```python
from build123d import *

# Parameters (mm, degrees)
BOSS_EXTRUDE1_DEPTH = 40
SKETCH3_R           = 1.5
CUT_EXTRUDE2_DEPTH  = 1
SKETCH4_R           = 1.5
SKETCH4_R_2         = 6
CUT_EXTRUDE3_DEPTH  = 10


with BuildPart() as part:
    # Sketch1 → Boss-Extrude1 (new body)
    with BuildSketch(Plane.XY):
        Polygon((0, 13), (0, 14), (7, 14), (11, 7.07179677), (10.133974596, 6.57179677), (6.422649731, 13), (1, 13), align=None)
    extrude(amount=BOSS_EXTRUDE1_DEPTH)

    # Sketch3 → Cut-Extrude2 (cut)
    with BuildSketch(Plane(origin=(11.312177826, 6.531088913, 0), x_dir=(0, 0, -1), z_dir=(0.8660254037844402, 0.4999999999999976, 0))):
        with Locations(Location((-36, 4.624355653, 0), (0, 0, 90))):
            Circle(SKETCH3_R)
        with Locations(Location((-4, 4.624355653, 0), (0, 0, 90))):
            Circle(SKETCH3_R)
        Polygon((-33.701530723, 0.624355653), (-27.721710311, 7.927360795), (-12.278289689, 7.927360795), (-6.298469277, 0.624355653), align=None)
    extrude(amount=-CUT_EXTRUDE2_DEPTH, mode=Mode.SUBTRACT)

    # Sketch4 → Cut-Extrude3 (cut)
    with BuildSketch(Plane(origin=(0, 14, 0), x_dir=(-1, 0, 0), z_dir=(0, 1, 0))):
        with Locations(Location((-3, 24.5, 0), (0, 0, 90))):
            Circle(SKETCH4_R)
        with Locations((4.185654705, 10)):
            Circle(SKETCH4_R_2)
        with Locations((4.185654705, 39)):
            Circle(SKETCH4_R_2)
    extrude(amount=-CUT_EXTRUDE3_DEPTH, mode=Mode.SUBTRACT)


solid = part.part
```
Source: CAD feature listing. Evaluate the final solid. Frame: model axes, mm. A direction names the side the tool comes from. Give positions to 0.01 mm unless a question says otherwise; leave off trailing zeros. Order: outer loops, then holes, each group sorted by start corner. A loop starts at its lowest first (then second) coordinate and runs counter-clockwise, first axis right, second up. Notation, with made-up numbers: (12, 10.5) -> (61, 10.5) arc R30 ccw to (61, 45.5) -> close; hole circle Ø10 at (1.5, 75.25). An arc over 180 degrees is marked (long way). Use a Markdown table: item, result.
Q1. Material intervals for line 1 (Y direction, x = 2.25, z = 34); line 2 (Z direction, x = 9.25, y = 9.75); line 3 (X direction, y = 13.7, z = 24.5), sorted ascending. Write a range as [from, to].
A:
| item | result |
|---|---|
| line 1 | [13, 14] |
| line 2 | [0, 2.73], [5.27, 8.91], [31.09, 34.73], [37.27, 40] |
| line 3 | [0, 1.5], [4.5, 7.17] |
Q2. Section A-A (z = 24.5). Return the cut outline in (x, y).
A:
| item | result |
|---|---|
| outline | (0, 13) -> (1.5, 13) -> (1.5, 14) -> (0, 14) -> close; (4.5, 13) -> (6.42, 13) -> (6.48, 12.9) -> (7.35, 13.4) -> (7, 14) -> (4.5, 14) -> close |
Q3. Pull-direction query (Z, two-part tool) for faces 4 (the face through (1.814, 13.507, 10.067)), 5 (the face through (7.4, 11.7, 40)), 6 (the face through (7.194, 13.664, 19.72)); classes: +Z half, -Z half, draft (parallel to the pull), parting line (faces both ways), or undercut.
A:
| item | result |
|---|---|
| face 4 | undercut |
| face 5 | +Z half |
| face 6 | draft |
Q4. Section C-C (x = 6). Return the cut outline in (y, z).
A:
| item | result |
|---|---|
| outline | (13, 0) -> (14, 0) -> (14, 40) -> (13, 40) -> close |
Q5. First-contact query: P1, Ø6, axis at x = 9, z = 23.5, coming from the +Y side; P2, Ø1, axis at y = 7.5, z = 4.5, coming from the -X side; P3, Ø2, axis at y = 12.5, z = 6, coming from the +X side; P4, Ø3, axis at x = 3.5, z = 19.5, coming from the -Y side. Flat tips, straight axial feed; report the tip coordinate or a pass-through.
A:
| item | result |
|---|---|
| P1 | y = 14 |
| P2 | x = 9.31 |
| P3 | x = 8.44 |
| P4 | y = 13 |
Q6. Section B-B (x = 3). Return the cut outline in (y, z), and give its area (3 significant figures).
A:
| item | result |
|---|---|
| outline | (13, 0) -> (14, 0) -> (14, 23) -> (13, 23) -> close; (13, 26) -> (14, 26) -> (14, 40) -> (13, 40) -> close |
| area | 37.0 mm^2 |
Q7. Access query for faces 1 (the face through (0, 13.5, 24.4)), 2 (the face through (8.72, 10.03, 9.33)), 3 (the face through (3, 13, 20)). Directions: +Z, -Z, +X, -X, +Y, -Y. A direction counts if a zero-diameter tool reaches every point of the face in a straight line with its end or side. Return the directions, or none.
A:
| item | result |
|---|---|
| face 1 | +Z, -Z, -X, +Y, -Y |
| face 2 | +X, -Y |
| face 3 | +Z, -Z, -X, -Y |
Q8. Section D-D (y = 9.25). State how many separate pieces and enclosed holes the cut face has, and give its area (3 significant figures).
A:
| item | result |
|---|---|
| separate pieces | 4 |
| enclosed holes | 0 |
| area | 15.9 mm^2 |
